Verification items for the finished model (mm, model axes). Give positions to 0.01 mm unless a question says otherwise; leave off trailing zeros. Order: outer loops, then holes, each group sorted by start corner. A loop starts at its lowest first (then second) coordinate and runs counter-clockwise, first axis right, second up.
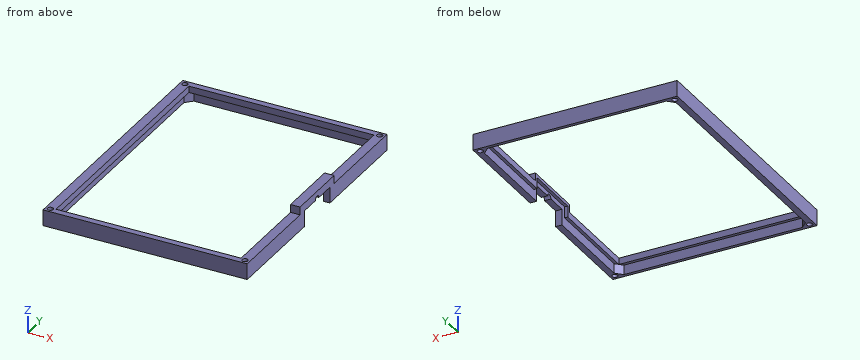
Autodesk Fusion 360 part; units mm, degrees
sketch "Sketch1" plane through (0, 0, 0) normal (0, 0, 1) x (1, 0, 0)
  line L0 (58, 78) -> (-58, 78)
  line L1 (-58, 78) -> (-58, -78)
  line L2 (-58, -78) -> (58, -78)
  line L3 (58, -78) -> (58, 78)
  line L4 (58, 78) -> (-58, -78) construction
  line L5 (-58, 78) -> (58, -78) construction
  circle A0 centre (-61, 79) radius 1.75
  line L6 (0, 2.5) -> (0, 20)
  circle A1 centre (61, 79) radius 1.75
  line L7 (20, 0) -> (2.5, 0)
  circle A2 centre (61, -79) radius 1.75
  circle A3 centre (-61, -79) radius 1.75
  line L8 (64, 82) -> (-64, 82)
  line L9 (-64, 82) -> (-64, -82)
  line L10 (-64, -82) -> (64, -82)
  line L11 (64, -82) -> (64, 82)
  line L12 (64, 82) -> (-64, -82) construction
  line L13 (-64, 82) -> (64, -82) construction
  dimension "d1" = 116
  dimension "d2" = 156
  dimension "d3" = 3.5
  dimension "d4" = 3
  dimension "d5" = 1
  dimension "d6" = 3
  dimension "d7" = 3
extrude "Extrude1" add sketch "Sketch1" along normal blind 10
sketch "Sketch2" plane through (0, 0, 0) normal (0, 0, 1) x (-1, 0, 0)
  line L0 (-58, -78) -> (-58, 78)
  line L1 (-58, 78) -> (58, 78)
  line L2 (58, 78) -> (58, -78)
  line L3 (58, -78) -> (-58, -78)
  circle A0 centre (-61, 79) radius 1.5
  circle A1 centre (-61, -79) radius 1.5
  circle A2 centre (61, 79) radius 1.5
  circle A3 centre (61, -79) radius 1.5
  line L4 (-64, 82) -> (-64, -82)
  line L5 (-64, -82) -> (64, -82)
  line L6 (64, -82) -> (64, 82)
  line L7 (64, 82) -> (-64, 82)
  line L8 (-60, 80) -> (60, 80)
  line L9 (60, 80) -> (60, -80)
  line L10 (60, -80) -> (-60, -80)
  line L11 (-60, -80) -> (-60, 80)
  line L12 (56, -80) -> (60, -76)
  line L13 (0, -2.5) -> (0, -20)
  line L14 (-56, -80) -> (-60, -76)
  line L15 (-20, 0) -> (-2.5, 0)
  line L16 (-56, 80) -> (-60, 76)
  line L17 (56, 80) -> (60, 76)
  line L18 (-58, 78) -> (-58, -78)
  line L19 (-58, -78) -> (58, -78)
  line L20 (58, -78) -> (58, 78)
  line L21 (58, 78) -> (-58, 78)
  circle A4 centre (-61, 79) radius 1.75
  circle A5 centre (-61, -79) radius 1.75
  circle A6 centre (61, 79) radius 1.75
  circle A7 centre (61, -79) radius 1.75
  line L22 (-64, -82) -> (-64, 82)
  line L23 (-64, 82) -> (64, 82)
  line L24 (64, 82) -> (64, -82)
  line L25 (64, -82) -> (-64, -82)
  dimension "d10" = -2
  dimension "d11" = 45
extrude "Extrude2" cut sketch "Sketch2" along normal blind 6 contours L0 L11 L14 L16 L18 | L3 L10 L12 L14 L19 | L1 L8 L16 L17 L21 | L2 L9 L12 L17 L20
sketch "Sketch3" plane through (0, 0, 0) normal (0, 0, 1) x (1, 0, 0)
  line L0 (58, 15) -> (64, 15)
  line L1 (64, 15) -> (64, -15)
  line L2 (64, -15) -> (58, -15)
  line L3 (58, -15) -> (58, 15)
  line L4 (64, -82) -> (64, 82)
  line L5 (58, -78) -> (58, 78)
  line L6 (58, 15) -> (64, 15)
  line L7 (64, 15) -> (64, 20)
  line L8 (64, 20) -> (58, 20)
  line L9 (58, 20) -> (58, 15)
  line L10 (58, -15) -> (64, -15)
  line L11 (64, -15) -> (64, -20)
  line L12 (64, -20) -> (58, -20)
  line L13 (58, -20) -> (58, -15)
  point P0 (58, 0)
  dimension "d14" = 30
  dimension "d15" = 5
  dimension "d16" = 5
extrude "Extrude3" add sketch "Sketch3" along normal blind 15
extrude "Extrude4" cut sketch "Sketch3" along normal blind 10 contours L0 L1 L2 L3 L4 L5 L6 L10
sketch "Sketch4" plane through (58, 0, 0) normal (-1, 0, 0) x (0, -1, 0)
  line L0 (-15, 0) -> (-15, 10)
  line L1 (-15, 10) -> (15, 10)
  line L2 (15, 10) -> (15, 0)
  line L3 (15, 0) -> (20, 0)
  line L4 (78, 6) -> (78, 10)
  line L5 (20, 6) -> (78, 6)
  line L6 (20, 0) -> (20, 6)
  line L7 (20, 15) -> (-20, 15)
  line L8 (-20, 15) -> (-20, 10)
  line L9 (-78, 10) -> (-78, 6)
  circle A0 centre (0, 10) radius 2
  line L10 (78, 10) -> (20, 10)
  line L11 (20, 10) -> (20, 15)
  line L12 (-20, 10) -> (-78, 10)
  line L13 (-78, 6) -> (-20, 6)
  line L14 (-20, 6) -> (-20, 0)
  line L15 (-20, 0) -> (-15, 0)
extrude "Extrude5" cut sketch "Sketch4" against normal blind 6 contours L1 A0 picked at (0.4887, 10.4534)
sketch "Sketch6" plane through (58, 0, 0) normal (-1, 0, 0) x (0, -1, 0)
  arc A0 (2, 10) -> (-2, 10) centre (0, 10) ccw
  line L0 (2, 10) -> (15, 10)
  line L1 (15, 10) -> (15, 0)
  line L2 (15, 0) -> (20, 0)
  line L3 (20, 0) -> (20, 6)
  line L4 (20, 6) -> (78, 6)
  line L5 (78, 6) -> (78, 10)
  line L6 (78, 10) -> (20, 10)
  line L7 (20, 10) -> (20, 15)
  line L8 (20, 15) -> (-20, 15)
  line L9 (-20, 15) -> (-20, 10)
  line L10 (-20, 10) -> (-78, 10)
  line L11 (-78, 10) -> (-78, 6)
  line L12 (-78, 6) -> (-20, 6)
  line L13 (-20, 6) -> (-20, 0)
  line L14 (-20, 0) -> (-15, 0)
  line L15 (-15, 0) -> (-15, 10)
  line L16 (-15, 10) -> (-2, 10)
  line L17 (-20, 6) -> (-18, 6)
  line L18 (-18, 6) -> (-18, 13)
  line L19 (-18, 13) -> (18, 13)
  line L20 (18, 13) -> (18, 6)
  line L21 (18, 6) -> (20, 6)
  dimension "d26" = 3
  dimension "d27" = 3
  dimension "d28" = 3
extrude "Extrude7" cut sketch "Sketch6" against normal blind 2 contours A0 L0 L1 L2 L3 L13 L14 L15 L16 L17 L18 L19 L20 L21
(1) Scan lines: line 1 (Y direction, x = 61, z = 3); line 2 (X direction, y = 79, z = 7.75); line 3 (Y direction, x = 42.5, z = 2.75). Record each from-to range of solid material in increasing order.
Solved:
line 1: y = -82 to -80.75, -77.25 to -15, 15 to 77.25, 80.75 to 82
line 2: x = -64 to -62.75, -59.25 to 59.25, 62.75 to 64
line 3: y = -82 to -80, 80 to 82
(2) Section check C-C, the plane z = 1.75. Enter the section's corners in (x, y).
Solved:
outline: (-64, -82) - (64, -82) - (64, -15) - (60, -15) - (60, -76) - (56, -80) - (-56, -80) - (-60, -76) - (-60, 76) - (-56, 80) - (56, 80) - (60, 76) - (60, 15) - (64, 15) - (64, 82) - (-64, 82) - close; hole circle Ø3.5 at (-61, -79); hole circle Ø3.5 at (-61, 79); hole circle Ø3.5 at (61, -79); hole circle Ø3.5 at (61, 79)
(3) Section check B-B, the plane y = 0. Enter the section's corners in (x, z), then the cut area to 3 significant figures.
Solved:
outline: (-64, 0) - (-60, 0) - (-60, 6) - (-58, 6) - (-58, 10) - (-64, 10) - close; (58, 13) - (60, 13) - (60, 12) - (64, 12) - (64, 15) - (58, 15) - close
area: 64.0 mm2
(4) Section check A-A, the plane x = 23.5. Enter the section's corners in (y, z), then the cut area to 3 significant figures.
Solved:
outline: (-82, 0) - (-80, 0) - (-80, 6) - (-78, 6) - (-78, 10) - (-82, 10) - close; (78, 6) - (80, 6) - (80, 0) - (82, 0) - (82, 10) - (78, 10) - close
area: 56.0 mm2
(5) Go/stop test with flat-tipped pins: pin 1 (1.6 mm diameter, centred on x = -19, y = -78.5, fed in from -Z); pin 2 (4.5 mm diameter, centred on x = 61, y = -79, fed in from +Z). Record where each tip stops, or that it passes through.
Solved:
pin 1: stops at z = 6
pin 2: stops at z = 10
